For this review, take the finished solid that the model builds, in its own axes (mm). Round coordinates to 2 decimals unless told otherwise and drop trailing zeros. Order: outer loops, then holes, each group sorted by start corner. A loop starts at its lowest first (then second) coordinate and runs counter-clockwise, first axis right, second up. Notation, with made-up numbers: (48.25, 29) -> (60.25, 29) arc R23 cw to (60.25, 49) -> close; hole circle Ø7 at (-9, 49). An arc over 180 degrees is marked (long way). Put each result on its own line as item: value. Start each with the question number.
```python
from build123d import *

# Parameters (mm, degrees)
BOSS_EXTRUDE1_DEPTH = 3
CUT_EXTRUDE1_REACH  = 242.652
SKETCH2_R           = 2.5
CUT_EXTRUDE2_REACH  = 242.652


with BuildPart() as part:
    # Sketch1 → Boss-Extrude1 (new body)
    with BuildSketch(Plane(origin=(0, 0, 0), x_dir=(0, 0, -1), z_dir=(1, 0, 0))):
        with BuildLine():
            Line((-12.188515962, 194.5), (106.683660563, 194.5))
            ThreePointArc((106.683660563, 194.5), (131.432397904, 184.248737342), (141.683660563, 159.5))
            Line((141.683660563, 159.5), (141.683660563, 20))
            ThreePointArc((141.683660563, 20), (131.432397904, -4.748737342), (106.683660563, -15))
            Line((106.683660563, -15), (-106.683660563, -15))
            ThreePointArc((-106.683660563, -15), (-128.230433314, -2.678193247), (-128.537592466, 22.141073279))
            Line((-128.537592466, 22.141073279), (-42.784020626, 176.497502591))
            ThreePointArc((-42.784020626, 176.497502591), (-29.937986507, 189.665481852), (-12.188515962, 194.5))
        make_face()
    extrude(amount=BOSS_EXTRUDE1_DEPTH)

    # Sketch2 → Cut-Extrude1 (cut, up to next)
    with BuildSketch(Plane(origin=(3, 0, 0), x_dir=(0, 0, -1), z_dir=(1, 0, 0)), mode=Mode.PRIVATE) as cut_extrude1_sk1:
        with Locations((81.683660563, 184.5)):
            Circle(SKETCH2_R)
    cut_extrude1_tool1 = extrude(cut_extrude1_sk1.sketch, amount=-CUT_EXTRUDE1_REACH, mode=Mode.PRIVATE) & part.part
    # Sketch2 → Cut-Extrude1 (cut, up to next)
    with BuildSketch(Plane(origin=(3, 0, 0), x_dir=(0, 0, -1), z_dir=(1, 0, 0)), mode=Mode.PRIVATE) as cut_extrude1_sk2:
        with Locations((12.811484038, 184.5)):
            Circle(SKETCH2_R)
    cut_extrude1_tool2 = extrude(cut_extrude1_sk2.sketch, amount=-CUT_EXTRUDE1_REACH, mode=Mode.PRIVATE) & part.part
    # Sketch2 → Cut-Extrude1 (cut, up to next)
    with BuildSketch(Plane(origin=(3, 0, 0), x_dir=(0, 0, -1), z_dir=(1, 0, 0)), mode=Mode.PRIVATE) as cut_extrude1_sk3:
        with Locations((131.683660563, 134.49995686)):
            Circle(SKETCH2_R)
    cut_extrude1_tool3 = extrude(cut_extrude1_sk3.sketch, amount=-CUT_EXTRUDE1_REACH, mode=Mode.PRIVATE) & part.part
    # Sketch2 → Cut-Extrude1 (cut, up to next)
    with BuildSketch(Plane(origin=(3, 0, 0), x_dir=(0, 0, -1), z_dir=(1, 0, 0)), mode=Mode.PRIVATE) as cut_extrude1_sk4:
        with Locations((131.683660563, 89.75)):
            Circle(SKETCH2_R)
    cut_extrude1_tool4 = extrude(cut_extrude1_sk4.sketch, amount=-CUT_EXTRUDE1_REACH, mode=Mode.PRIVATE) & part.part
    # Sketch2 → Cut-Extrude1 (cut, up to next)
    with BuildSketch(Plane(origin=(3, 0, 0), x_dir=(0, 0, -1), z_dir=(1, 0, 0)), mode=Mode.PRIVATE) as cut_extrude1_sk5:
        with Locations((131.683660563, 44.999939605)):
            Circle(SKETCH2_R)
    cut_extrude1_tool5 = extrude(cut_extrude1_sk5.sketch, amount=-CUT_EXTRUDE1_REACH, mode=Mode.PRIVATE) & part.part
    # Sketch2 → Cut-Extrude1 (cut, up to next)
    with BuildSketch(Plane(origin=(3, 0, 0), x_dir=(0, 0, -1), z_dir=(1, 0, 0)), mode=Mode.PRIVATE) as cut_extrude1_sk6:
        with Locations((71.683660563, -5)):
            Circle(SKETCH2_R)
    cut_extrude1_tool6 = extrude(cut_extrude1_sk6.sketch, amount=-CUT_EXTRUDE1_REACH, mode=Mode.PRIVATE) & part.part
    # Sketch2 → Cut-Extrude1 (cut, up to next)
    with BuildSketch(Plane(origin=(3, 0, 0), x_dir=(0, 0, -1), z_dir=(1, 0, 0)), mode=Mode.PRIVATE) as cut_extrude1_sk7:
        with Locations((0, -5)):
            Circle(SKETCH2_R)
    cut_extrude1_tool7 = extrude(cut_extrude1_sk7.sketch, amount=-CUT_EXTRUDE1_REACH, mode=Mode.PRIVATE) & part.part
    # Sketch2 → Cut-Extrude1 (cut, up to next)
    with BuildSketch(Plane(origin=(3, 0, 0), x_dir=(0, 0, -1), z_dir=(1, 0, 0)), mode=Mode.PRIVATE) as cut_extrude1_sk8:
        with Locations((-71.683660563, -5)):
            Circle(SKETCH2_R)
    cut_extrude1_tool8 = extrude(cut_extrude1_sk8.sketch, amount=-CUT_EXTRUDE1_REACH, mode=Mode.PRIVATE) & part.part
    # Sketch2 → Cut-Extrude1 (cut, up to next)
    with BuildSketch(Plane(origin=(3, 0, 0), x_dir=(0, 0, -1), z_dir=(1, 0, 0)), mode=Mode.PRIVATE) as cut_extrude1_sk9:
        with Locations((-100.370302458, 52.250935013)):
            Circle(SKETCH2_R)
    cut_extrude1_tool9 = extrude(cut_extrude1_sk9.sketch, amount=-CUT_EXTRUDE1_REACH, mode=Mode.PRIVATE) & part.part
    # Sketch2 → Cut-Extrude1 (cut, up to next)
    with BuildSketch(Plane(origin=(3, 0, 0), x_dir=(0, 0, -1), z_dir=(1, 0, 0)), mode=Mode.PRIVATE) as cut_extrude1_sk10:
        with Locations((-76.919233785, 94.462858624)):
            Circle(SKETCH2_R)
    cut_extrude1_tool10 = extrude(cut_extrude1_sk10.sketch, amount=-CUT_EXTRUDE1_REACH, mode=Mode.PRIVATE) & part.part
    # Sketch2 → Cut-Extrude1 (cut, up to next)
    with BuildSketch(Plane(origin=(3, 0, 0), x_dir=(0, 0, -1), z_dir=(1, 0, 0)), mode=Mode.PRIVATE) as cut_extrude1_sk11:
        with Locations((-53.468165112, 136.674782235)):
            Circle(SKETCH2_R)
    cut_extrude1_tool11 = extrude(cut_extrude1_sk11.sketch, amount=-CUT_EXTRUDE1_REACH, mode=Mode.PRIVATE) & part.part
    add(cut_extrude1_tool1.solids().sort_by_distance((3, 184.5, -81.683661))[0], mode=Mode.SUBTRACT)
    add(cut_extrude1_tool2.solids().sort_by_distance((3, 184.5, -12.811484))[0], mode=Mode.SUBTRACT)
    add(cut_extrude1_tool3.solids().sort_by_distance((3, 134.499957, -131.683661))[0], mode=Mode.SUBTRACT)
    add(cut_extrude1_tool4.solids().sort_by_distance((3, 89.75, -131.683661))[0], mode=Mode.SUBTRACT)
    add(cut_extrude1_tool5.solids().sort_by_distance((3, 44.99994, -131.683661))[0], mode=Mode.SUBTRACT)
    add(cut_extrude1_tool6.solids().sort_by_distance((3, -5, -71.683661))[0], mode=Mode.SUBTRACT)
    add(cut_extrude1_tool7.solids().sort_by_distance((3, -5, 0))[0], mode=Mode.SUBTRACT)
    add(cut_extrude1_tool8.solids().sort_by_distance((3, -5, 71.683661))[0], mode=Mode.SUBTRACT)
    add(cut_extrude1_tool9.solids().sort_by_distance((3, 52.250935, 100.370302))[0], mode=Mode.SUBTRACT)
    add(cut_extrude1_tool10.solids().sort_by_distance((3, 94.462859, 76.919234))[0], mode=Mode.SUBTRACT)
    add(cut_extrude1_tool11.solids().sort_by_distance((3, 136.674782, 53.468165))[0], mode=Mode.SUBTRACT)

    # Sketch3 → Cut-Extrude2 (cut, up to next)
    with BuildSketch(Plane(origin=(3, 0, 0), x_dir=(0, 0, -1), z_dir=(1, 0, 0)), mode=Mode.PRIVATE) as cut_extrude2_sk1:
        with BuildLine():
            Line((71.683660563, 159.5), (71.683660563, 194.5))
            Line((71.683660563, 194.5), (106.683660563, 194.5))
            ThreePointArc((106.683660563, 194.5), (131.432397904, 184.248737342), (141.683660563, 159.5))
            Line((141.683660563, 159.5), (141.683660563, 124.5))
            Line((141.683660563, 124.5), (106.683660563, 124.5))
            ThreePointArc((106.683660563, 124.5), (81.934923221, 134.751262658), (71.683660563, 159.5))
        make_face()
    cut_extrude2_tool1 = extrude(cut_extrude2_sk1.sketch, amount=-CUT_EXTRUDE2_REACH, mode=Mode.PRIVATE) & part.part
    add(cut_extrude2_tool1.solids().sort_by_distance((3, 159.5, -106.683661))[0], mode=Mode.SUBTRACT)


solid = part.part
```
Item 1: Insertion check: pin 1 Ø2 at (y, z) = (79, -110) entering from -X; pin 2 Ø1.5 at (x, z) = (2, -122.5) entering from +Y; pin 3 Ø0.9 at (x, y) = (1, 176.5) entering from -Z. Each pin has a flat end and moves straight along its axis. Give the tip position at first contact, or say it passes through.
Item 2: For L1, parallel to Y at x = 2.3, z = 75; L2, parallel to Y at x = 0.65, z = 39; L3, parallel to Y at x = 1.95, z = -108, list the stretches that pass through material, from the lowest coordinate up.
Item 3: Consider section C-C, the plane y = 0.5. Write out the cut boundary in (x, z).
Item 4: Consider section B-B, the plane y = 76. Write out the cut boundary in (x, z), plus the area to 3 significant figures.
Item 5: Consider section A-A, the plane x = 0.65. Count the separate pieces of the cut face and the enclosed holes in it, plus the area to 3 significant figures.
Evaluation:
1. pin 1: stops at x = 0
1. pin 2: stops at y = 124.5
1. pin 3: stops at z = -71.68
2. L1: y = -15 to 92.86, 96.06 to 118.51
2. L2: y = -15 to 182
2. L3: y = -14.98 to 124.5
3. outline: (0, -135.75) -> (3, -135.75) -> (3, 129.81) -> (0, 129.81) -> close
4. outline: (0, -141.68) -> (3, -141.68) -> (3, 98.62) -> (0, 98.62) -> close
4. area: 721 mm^2
5. separate pieces: 1
5. enclosed holes: 9
5. area: 43,200 mm^2
